```python
from build123d import *

# Parameters (mm, degrees)
SKETCH1_W               = 25.267998504
SKETCH1_H               = 2.54
BOSS_EXTRUDE7_DEPTH     = 9.144
BOSS_EXTRUDE9_START     = -2.032
BOSS_EXTRUDE9_OUTLINE_W = 4.303574795
BOSS_EXTRUDE9_OUTLINE_H = 4.327328355
BOSS_EXTRUDE9_DEPTH     = 2.032


# Read off the part's stored shape, not the designer's step: Boss-Extrude9
with BuildPart() as part:
    # Sketch1 → Boss-Extrude7 (new body)
    # profile 1 of 5: a face of its own
    with BuildSketch(Plane(origin=(0, 0, 0), x_dir=(1, 0, 0), z_dir=(0, 1, 0))):
        with BuildLine():
            ThreePointArc((20.091392362, -14.973938339), (36.674866164, -15.633001334), (38.077226225, 0.904209847))
            ThreePointArc((38.077226225, 0.904209847), (36.965236291, 17.810596862), (20.053933255, 16.7760568))
            Line((20.053933255, 16.7760568), (-15.464178996, 16.7760568))
            ThreePointArc((-15.464178996, 16.7760568), (-32.391267437, 17.810916917), (-33.472263124, 0.886712153))
            ThreePointArc((-33.472263124, 0.886712153), (-32.31789128, -15.981799893), (-15.439991882, -14.973938339))
            Line((-15.439991882, -14.973938339), (20.091392362, -14.973938339))
        make_face()
        with BuildLine():
            ThreePointArc((-29.65629843, 0.90105923), (-31.167264268, -13.573979358), (-16.658299233, -12.433938339))
            Line((-16.658299233, -12.433938339), (21.246557929, -12.433938339))
            ThreePointArc((21.246557929, -12.433938339), (35.496314389, -13.251428184), (34.363784281, 0.976755972))
            ThreePointArc((34.363784281, 0.976755972), (35.768086185, 15.449459714), (21.2781286, 14.2360568))
            Line((21.2781286, 14.2360568), (-16.689869904, 14.2360568))
            ThreePointArc((-16.689869904, 14.2360568), (-31.234591455, 15.407251461), (-29.65629843, 0.90105923))
        make_face(mode=Mode.SUBTRACT)
    # profile 2 of 5: a face of its own
    with BuildSketch(Plane(origin=(0, 0, 0), x_dir=(1, 0, 0), z_dir=(0, 1, 0))):
        with BuildLine():
            ThreePointArc((-33.474089865, -4.305938339), (-28.507587271, -15.489738966), (-16.658299233, -12.433938339))
            Line((-16.658299233, -12.433938339), (-10.339869904, -12.433938339))
            Line((-10.339869904, -12.433938339), (-10.339869904, -9.893938339))
            Line((-10.339869904, -9.893938339), (-16.658299233, -9.893938339))
            Line((-16.658299233, -9.893938339), (-23.008299233, -9.893938339))
            Line((-23.008299233, -9.893938339), (-23.008299233, -4.305938339))
            Line((-23.008299233, -4.305938339), (-33.474089865, -4.305938339))
        make_face()
    # profile 3 of 5: a face of its own
    with BuildSketch(Plane(origin=(0, 0, 0), x_dir=(1, 0, 0), z_dir=(0, 1, 0))):
        with Locations((2.294129348, -11.163938339)):
            Rectangle(SKETCH1_W, SKETCH1_H)
    # profile 4 of 5: a face of its own
    with BuildSketch(Plane(origin=(0, 0, 0), x_dir=(1, 0, 0), z_dir=(0, 1, 0))):
        with BuildLine():
            Line((14.9281286, -9.893938339), (14.9281286, -12.433938339))
            Line((14.9281286, -12.433938339), (21.246557929, -12.433938339))
            ThreePointArc((21.246557929, -12.433938339), (35.496314389, -13.251428184), (34.363784281, 0.976755972))
            Line((34.363784281, 0.976755972), (26.449874225, 0.976755972))
            Line((26.449874225, 0.976755972), (26.449874225, -9.893938339))
            Line((26.449874225, -9.893938339), (21.246557929, -9.893938339))
            Line((21.246557929, -9.893938339), (14.9281286, -9.893938339))
        make_face()
    # profile 5 of 5: a face of its own
    with BuildSketch(Plane(origin=(0, 0, 0), x_dir=(1, 0, 0), z_dir=(0, 1, 0))):
        with Locations((2.294129348, 12.9660568)):
            Rectangle(SKETCH1_W, SKETCH1_H)
    extrude(amount=BOSS_EXTRUDE7_DEPTH)

    # Boss-Extrude9 outline → Boss-Extrude9 (add)
    with BuildSketch(Plane(origin=(0, 0, 2.54), x_dir=(-1, 0, 0), z_dir=(0, 1, 0)).offset(BOSS_EXTRUDE9_START)):
        with BuildLine():
            ThreePointArc((-39.962274592, 8.331071624), (-40.584803359, 2.192889064), (-38.077226225, -3.444209847))
            ThreePointArc((-38.077226225, -3.444209847), (-39.980253201, -6.412725487), (-40.938977335, -9.806019581))
            ThreePointArc((-40.938977335, -9.806019581), (-34.00622148, -22.23363184), (-20.077959401, -19.316070247))
            Line((-20.077959401, -19.316070247), (-20.053939231, -19.316070247))
            Line((-20.053939231, -19.316070247), (15.464178996, -19.3160568))
            ThreePointArc((15.464178996, -19.3160568), (16.013662974, -19.895397798), (16.600434504, -20.436939861))
            ThreePointArc((16.600434504, -20.436939861), (32.922411354, -19.767481007), (33.473277412, -3.441071419))
            ThreePointArc((33.473277412, -3.441071419), (33.476154659, -3.437751763), (33.47903069, -3.434431054))
            ThreePointArc((33.47903069, -3.434431054), (33.475647732, -3.43057088), (33.472263124, -3.426712153))
            ThreePointArc((33.472263124, -3.426712153), (35.310098705, 9.413648761), (24.402438556, 16.433296764))
            ThreePointArc((24.402438556, 16.433296764), (19.501273126, 15.38830994), (15.453425616, 12.433931737))
            Line((15.453425616, 12.433931737), (-20.091392362, 12.433938339))
            ThreePointArc((-20.091392362, 12.433938339), (-22.408655082, 14.301808135), (-25.114144013, 15.542361937))
            ThreePointArc((-25.114144013, 15.542361937), (-33.970966426, 14.886780351), (-39.962274592, 8.331071624))
        make_face()
        with Locations((-29.515589711, -13.831402182)):
            Rectangle(BOSS_EXTRUDE9_OUTLINE_W, BOSS_EXTRUDE9_OUTLINE_H, mode=Mode.SUBTRACT)
        with Locations((24.644768928, -13.703519078)):
            Rectangle(BOSS_EXTRUDE9_OUTLINE_W, BOSS_EXTRUDE9_OUTLINE_H, mode=Mode.SUBTRACT)
        Polygon((32.612403312, 1.632473231), (32.612403312, -1.682770742), (20.573249237, -1.682770742), (20.573249237, -8.754579205), (16.565180299, -8.754579205), (16.565180299, 0.209107335), (20.573249237, 0.209107335), (20.573249237, 1.632473231), align=None, mode=Mode.SUBTRACT)
    extrude(amount=BOSS_EXTRUDE9_DEPTH)


solid = part.part
```
Verification items for the finished model (mm, model axes). A direction names the side the tool comes from. Give positions to 0.01 mm unless a question says otherwise; leave off trailing zeros. Return JSON: item names as keys, results as strings.
1) Section check A-A, the plane y = -1. Count the separate pieces of the cut face and the enclosed holes in it, and give its area (3 significant figures).
Findings:
{"separate pieces": "1", "enclosed holes": "3", "area": "2,470 mm2"}
2) Material ranges on L1, parallel to Z at x = -3.5, y = 3; L2, parallel to Z at x = -24, y = 8; L3, parallel to X at y = 6.75, z = -17, recorded low to high. Write a range as [from, to].
Findings:
{"L1": "z = [-16.78, -11.7], [9.89, 14.97]", "L2": "z = [-20.81, -18.26], [4.31, 18.97]", "L3": "x = [-33.23, -29.19], [-19.7, -15.67], [20.26, 24.3], [33.76, 37.8]"}
3) Gauge pin test, flat ends, axial feed: P1, Ø2, axis at y = -0.5, z = -4, coming from the +X side; P2, Ø4, axis at x = -3.5, y = 3.5, coming from the -Z side; P3, Ø22.5, axis at x = 1.5, z = -6, coming from the +Y side; P4, Ø1.7, axis at y = 6.5, z = 7.5, coming from the +X side. Record the tip position at first contact, or that the pin passes through.
Findings:
{"P1": "stops at x = 40.42", "P2": "stops at z = -16.78", "P3": "stops at y = 9.14", "P4": "stops at x = 40.74"}
4) Mould release check, pull along X, two halves, no side actions. Record for faces 1 (the flat face through (2, 9.144, 11)), 2 (the flat face through (-32.612, -1, 3)): released by +X, released by -X, zero draft, split by the parting line, or undercut.
Findings:
{"face 1": "zero draft", "face 2": "undercut"}
5) Tool access check on faces 3 (the cylindrical face through (-32.743, -1.03, -17.404)), 4 (the flat face through (2, 5, 14.974)), 5 (the flat face through (31.667, -1, -11)). Record the directions out of +Z, -Z, +X, -X, +Y, -Y that give a thin tool (end or side, any length) a straight path to the whole face; none if there is none.
Findings:
{"face 3": "-Y", "face 4": "+Z, +Y, -Y", "face 5": "+Y, -Y"}
